from build123d import *

# Parameters (mm, degrees)
SKETCH2_R          = 2.6
BASE_FLANGE1_DEPTH = 6
FILLET1_R          = 5
FILLET2_R          = 2
SKETCH6_R          = 3
SKETCH6_W          = 6.9
SKETCH6_H          = 10.3
SKETCH6_W_2        = 10.3
SKETCH6_H_2        = 6.9
CUT_EXTRUDE3_DEPTH = 10


# Sheet-metal steps are written as plain solids
with BuildPart() as part:
    # Sketch2 → Base-Flange1 (new body)
    with BuildSketch(Plane(origin=(0, 0, 0), x_dir=(1, 0, 0), z_dir=(0, 1, 0))):
        Polygon((0, 72), (65, 72), (65, 5), (20, 5), (20, 25), (0, 25), align=None)
        with Locations(Location((28, 9, 0), (0, 0, 270))):
            Circle(SKETCH2_R, mode=Mode.SUBTRACT)
        with Locations(Location((43, 9, 0), (0, 0, 270))):
            Circle(SKETCH2_R, mode=Mode.SUBTRACT)
        with Locations(Location((58, 9, 0), (0, 0, 270))):
            Circle(SKETCH2_R, mode=Mode.SUBTRACT)
        with Locations(Location((9, 33, 0), (0, 0, 270))):
            Circle(SKETCH2_R, mode=Mode.SUBTRACT)
        with Locations(Location((9, 48, 0), (0, 0, 270))):
            Circle(SKETCH2_R, mode=Mode.SUBTRACT)
        with Locations(Location((9, 63, 0), (0, 0, 270))):
            Circle(SKETCH2_R, mode=Mode.SUBTRACT)
    extrude(amount=-BASE_FLANGE1_DEPTH)

    # Fillet1
    fillet1_edges = [part.edges().sort_by_distance(p)[0] for p in [
        (0, -3, -25),
        (0, -3, -72),
        (65, -3, -72),
        (65, -3, -5),
        (20, -3, -5),
    ]]
    fillet(fillet1_edges, radius=FILLET1_R)

    # Fillet2
    fillet2_edges = [part.edges().sort_by_distance(p)[0] for p in [
        (20, -3, -25),
    ]]
    fillet(fillet2_edges, radius=FILLET2_R)

    # Sketch6 → Cut-Extrude3 (cut)
    with BuildSketch(Plane(origin=(0, 0, 0), x_dir=(1, 0, 0), z_dir=(0, 1, 0))):
        with Locations(Location((43, 48, 0), (0, 0, 270))):
            Circle(SKETCH6_R)
        with Locations((27, 48)):
            Rectangle(SKETCH6_W, SKETCH6_H)
        with Locations((43, 31)):
            Rectangle(SKETCH6_W_2, SKETCH6_H_2)
        with Locations((43, 65)):
            Rectangle(SKETCH6_W_2, SKETCH6_H_2)
    extrude(amount=-CUT_EXTRUDE3_DEPTH, mode=Mode.SUBTRACT)


solid = part.part
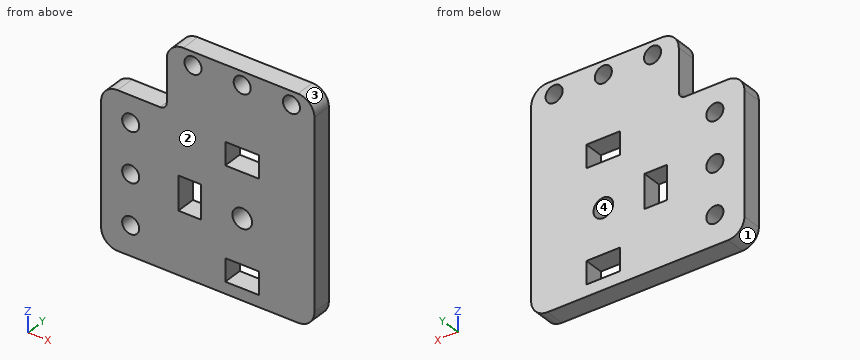
Can you work these out from the model? Positions are in its coordinate system, mm. Face numbers are marked on the shaded views. Coordinates: 2 decimals unless noted, no trailing zeros. Order: outer loops, then holes, each group sorted by start corner. A loop starts at its lowest first (then second) coordinate and runs counter-clockwise, first axis right, second up. Notation, with made-up numbers: (-22.5, 66) -> (-15.5, 66) arc R25 cw to (-15.5, 86) -> close; hole circle Ø10 at (44, 58). An arc over 180 degrees is marked (long way). Use one line per item in the form item = value.
Q1. We'd pull the mould along X, two halves only. Please class the marked faces 1, 2, 3 and 4: released by +X, released by -X, zero draft, split by the parting line, or undercut.
From the geometry:
face_1 = released by -X
face_2 = zero draft
face_3 = released by +X
face_4 = undercut
Q2. Imagine slicing it at C-C, the plane y = -2.65. Give the number of separate pieces and of enclosed holes in the cut face, then the cut area to 3 significant figures.
From the geometry:
separate_pieces = 1
enclosed_holes = 10
area = 3,560 mm²
Q3. Will this pin go through, and if not, where does the flat tip stop? P1, Ø3, axis at y = -4, z = -14, coming from the -X side.
From the geometry:
P1 = 20
Q4. Imagine slicing it at B-B, the plane z = -63. List the corners of the cut face in (x, y) for me.
From the geometry:
outline = (0, -6) -> (6.4, -6) -> (6.4, 0) -> (0, 0) -> close; (11.6, -6) -> (37.85, -6) -> (37.85, 0) -> (11.6, 0) -> close; (48.15, -6) -> (65, -6) -> (65, 0) -> (48.15, 0) -> close
Q5. Imagine slicing it at A-A, the plane x = 58. List the corners of the cut face in (y, z) for me.
From the geometry:
outline = (-6, -72) -> (0, -72) -> (0, -11.6) -> (-6, -11.6) -> close; (-6, -6.4) -> (0, -6.4) -> (0, -5) -> (-6, -5) -> close
Q6. I need wall thicknesses on L1, parallel to X at y = -4, z = -63; L2, parallel to Z at x = 47, y = -3.15; L3, parallel to Z at x = 7.5, y = -4.8. Which ranges of each line are inside material? Lowest first, please.
From the geometry:
L1 = 0 to 6.4, 11.6 to 37.85, 48.15 to 65
L2 = -72 to -68.45, -61.55 to -34.45, -27.55 to -5
L3 = -72 to -65.12, -60.88 to -50.12, -45.88 to -35.12, -30.88 to -25
Q7. Imagine slicing it at D-D, the plane x = 43. List the corners of the cut face in (y, z) for me.
From the geometry:
outline = (-6, -72) -> (0, -72) -> (0, -68.45) -> (-6, -68.45) -> close; (-6, -61.55) -> (0, -61.55) -> (0, -51) -> (-6, -51) -> close; (-6, -45) -> (0, -45) -> (0, -34.45) -> (-6, -34.45) -> close; (-6, -27.55) -> (0, -27.55) -> (0, -11.6) -> (-6, -11.6) -> close; (-6, -6.4) -> (0, -6.4) -> (0, -5) -> (-6, -5) -> close
